from build123d import *

# Parameters (mm, degrees)
F0_R     = 3.354118
F1_DEPTH = 6.35
F2_R     = 1.499831
F3_DEPTH = 97.282
F4_R     = 1.083943
F5_DEPTH = 20.574


with BuildPart() as f1:
    # F0 (on Front) → F1 (new body)
    with BuildSketch(Plane.XZ):
        with Locations((-35.692804, 10.552901)):
            Circle(F0_R)
    extrude(amount=F1_DEPTH)

    # F2 (on Front) → F3 (join)
    with BuildSketch(Plane.XZ):
        with Locations((-35.80986, 10.426732)):
            Circle(F2_R)
    extrude(amount=-F3_DEPTH)

    # F4 (on Front) → F5 (join)
    with BuildSketch(Plane.XZ):
        with Locations((-35.32517, 10.668001)):
            Circle(F4_R)
    extrude(amount=-F5_DEPTH)


solid = f1.part
Model file for the job. Use its own axes, mm. A direction names the side the tool comes from. Coordinates: 2 decimals unless noted, no trailing zeros. Order: outer loops, then holes, each group sorted by start corner. A loop starts at its lowest first (then second) coordinate and runs counter-clockwise, first axis right, second up. Notation, with made-up numbers: (39.5, -37) -> (88.5, -37) arc R25 cw to (88.5, -6) -> close; hole circle Ø10 at (83, -20). An arc over 180 degrees is marked (long way). Return JSON: item names as keys, results as strings. Group by question number.
Item 1: Flat gauge pins, fed straight in: P1, Ø2, axis at x = -33, z = 10.5, coming from the +Y side; P2, Ø2, axis at y = 37.5, z = 9.5, coming from the -X side; P3, Ø2, axis at y = 63, z = 12.5, coming from the +X side; P4, Ø2, axis at x = -36.5, z = 12, coming from the +Y side. Where does each tip first touch, or does it go through?
Item 2: Saw through at D-D on y = 59.5. Write the cut outline in (x, z).
Item 3: Tool access for faces 1 (the flat face through (-36, 97.282, 10)), 2 (the flat face through (-34, 0, 10)): list every direction of +Z, -Z, +X, -X, +Y, -Y with a clear straight run to the whole face (end or side of a thin tool).
Item 4: Saw through at C-C on y = 14.5. Write the cut outline in (x, z), then the cut area to 3 significant figures.
Item 5: Wall check: line 1 along Y through (x, z) = (-38, 11.75); line 2 along Z through (x, y) = (-36, 36); line 3 along Z through (x, y) = (-34.75, 57). Give the ranges that are in metal, low to high. Write a range as [from, to].
Item 6: Saw through at B-B on z = 13. Write the cut outline in (x, y).
Item 7: Saw through at A-A on x = -36.25. Write the cut outline in (y, z), then the cut area to 3 significant figures.
Values found:
{
 "1": {"P1": "stops at y = 0", "P2": "stops at x = -37.31", "P3": "stops at x = -34.76", "P4": "stops at y = 97.28"},
 "2": {"outline": "circle Ø3 at (-35.81, 10.43)"},
 "3": {"face 1": "+Z, -Z, +X, -X, +Y", "face 2": "+Y"},
 "4": {"outline": "(-35.04, 11.71) arc R1.5 ccw (long way) to (-34.32, 10.27) arc R1.08 ccw to start", "area": "7.21 mm2"},
 "5": {"line 1": "y = [-6.35, 0]", "line 2": "z = [8.94, 11.91]", "line 3": "z = [9.37, 11.49]"},
 "6": {"outline": "(-37.99, -6.35) -> (-33.4, -6.35) -> (-33.4, 0) -> (-37.99, 0) -> close"},
 "7": {"outline": "(-6.35, 7.25) -> (0, 7.25) -> (0, 8.99) -> (97.28, 8.99) -> (97.28, 11.86) -> (0, 11.86) -> (0, 13.86) -> (-6.35, 13.86) -> close", "area": "321 mm2"}
}
